The model under review builds one solid part; all positions refer to its coordinate system, in mm. Face numbers are marked on the shaded views. A direction names the side the tool comes from. Round coordinates to 2 decimals unless told otherwise and drop trailing zeros. Loops run counter-clockwise (first coordinate to the right, second up) from the corner with the lowest first, then second, coordinate; pieces in that order, holes last. Notation, with made-up numbers: (-11, 53.5) -> (37, 53.5) arc R24 ccw to (37, 69.5) -> close; hole circle Ø7 at (54.25, -38). An arc over 180 degrees is marked (long way). Write each question's results on one line, items separated by ' | '. Start each with the question number.
Item 1: Clearance check with flat-ended pins moving along their axes: pin 1 Ø5 at (y, z) = (-55.5, -13) entering from +X; pin 2 Ø8 at (x, y) = (-30, -45) entering from -Z; pin 3 Ø2 at (y, z) = (-78.5, 4.5) entering from -X. State where each tip first meets the part, or that it passes through.
Item 2: For L1, parallel to Z at x = 0, y = -58.5; L2, parallel to Z at x = 0, y = -39; L3, parallel to Y at x = 36, z = -21, list the stretches that pass through material, from the lowest coordinate up. Write a range as from..to.
Item 3: Tool access review of the marked faces 1 and 2: name each direction out of +Z, -Z, +X, -X, +Y, -Y from which nothing blocks a thin tool from reaching the whole face with its end or side.
Item 4: We need section C-C (x = 0). Give the boundary of the cut face in (y, z), and give its area (3 significant figures).
Item 5: We need section A-A (z = 0). Give the boundary of the cut face in (x, y).
Item 6: Mouldability with a two-part tool opening along X and no side actions: class the marked faces 3, 4 and 5 as pulls with the +X half, pulls with the -X half, needs draft (parallel to the pull), parting line crosses it, or undercut.
Item 7: We need section B-B (y = -34). Give the boundary of the cut face in (x, z).
Item 8: We need section D-D (y = -44.5). Give the boundary of the cut face in (x, z).
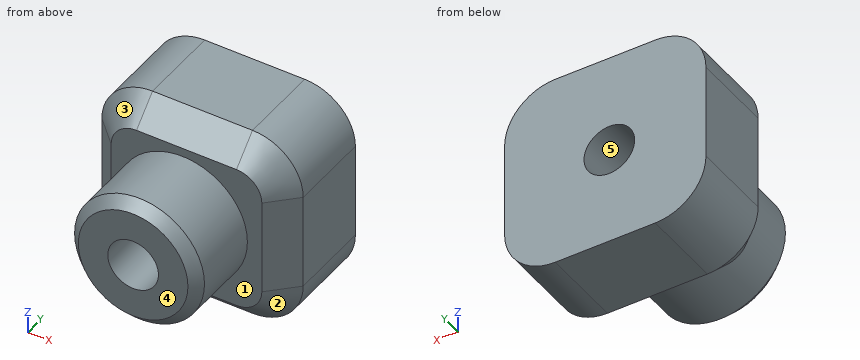
from build123d import *

# Parameters (mm, degrees)
F0_W     = 100.887247
F0_H     = 98.669946
F1_DEPTH = 53.981356
F2_R     = 25.4
F3_R     = 32.544511
F4_DEPTH = 39.004393
F6_D     = 25.4
F7_SIZE  = 12.7
F8_SIZE  = 5.08


with BuildPart() as f1:
    # F0 (on Front) → F1 (new body)
    with BuildSketch(Plane.XZ):
        with Locations((2.032529, 0.184774)):
            Rectangle(F0_W, F0_H)
    extrude(amount=F1_DEPTH)

    # F2
    f2_edges = [f1.edges().sort_by_distance(p)[0] for p in [
        (52.476153, -26.990678, 49.519747),
        (52.476153, -26.990678, -49.150199),
        (-48.411094, -26.990678, -49.150199),
        (-48.411094, -26.990678, 49.519747),
    ]]
    fillet(f2_edges, radius=F2_R)

    # F3 (on face) → F4 (join)
    with BuildSketch(Plane.XZ.offset(53.981356)):
        Circle(F3_R)
    extrude(amount=F4_DEPTH)

    # F6 (through all)
    with Locations(Plane.XZ.offset(92.985749)):
        with Locations((0, 0)):
            Hole(F6_D / 2)

    # F7
    f7_edges = [f1.edges().sort_by_distance(p)[0] for p in [
        (-48.411094, -53.981356, 0.184774),
    ]]
    chamfer(f7_edges, length=F7_SIZE)

    # F8
    f8_edges = [f1.edges().sort_by_distance(p)[0] for p in [
        (-32.544511, -92.985749, 0),
    ]]
    chamfer(f8_edges, length=F8_SIZE)


solid = f1.part
Here are the results:
1) pin 1: stops at x = 40.76 | pin 2: stops at z = -48.54 | pin 3: stops at x = -32.36
2) L1: z = -32.54..-12.7, 12.7..32.54 | L2: z = -49.15..-12.7, 12.7..49.52 | L3: y = -53.98..0
3) face 1: -Y | face 2: -Z, +X, -Y
4) outline: (-92.99, -27.46) -> (-87.91, -32.54) -> (-53.98, -32.54) -> (-53.98, -36.45) -> (-41.28, -49.15) -> (0, -49.15) -> (0, -12.7) -> (-92.99, -12.7) -> close; (-92.99, 12.7) -> (0, 12.7) -> (0, 49.52) -> (-41.28, 49.52) -> (-53.98, 36.82) -> (-53.98, 32.54) -> (-87.91, 32.54) -> (-92.99, 27.46) -> close | area: 5,320 mm2
5) outline: (-48.41, -41.28) -> (-35.71, -53.98) -> (-32.54, -53.98) -> (-32.54, -87.91) -> (-27.46, -92.99) -> (-12.7, -92.99) -> (-12.7, 0) -> (-48.41, 0) -> close; (12.7, -92.99) -> (27.46, -92.99) -> (32.54, -87.91) -> (32.54, -53.98) -> (39.78, -53.98) -> (52.48, -41.28) -> (52.48, 0) -> (12.7, 0) -> close
6) face 3: pulls with the -X half | face 4: needs draft | face 5: undercut
7) outline: (-48.41, -23.75) arc R25.4 ccw to (-23.01, -49.15) -> (27.08, -49.15) arc R25.4 ccw to (52.48, -23.75) -> (52.48, 24.12) arc R25.4 ccw to (27.08, 49.52) -> (-23.01, 49.52) arc R25.4 ccw to (-48.41, 24.12) -> close; hole circle Ø25.4 at (0, 0)
8) outline: (-45.19, -23.75) arc R22.18 ccw to (-23.01, -45.93) -> (27.08, -45.93) arc R22.18 ccw to (49.26, -23.75) -> (49.26, 24.12) arc R22.18 ccw to (27.08, 46.3) -> (-23.01, 46.3) arc R22.18 ccw to (-45.19, 24.12) -> close; hole circle Ø25.4 at (0, 0)
